Job drawing, mm, ordinate dimensions from the low corner. One solid piece. A direction names the side the tool comes from. Coordinates: 2 decimals unless noted, no trailing zeros. Order: outer loops, then holes, each group sorted by start corner. A loop starts at its lowest first (then second) coordinate and runs counter-clockwise, first axis right, second up. Notation, with made-up numbers: (-21, 52) -> (1, 52) arc R16 ccw to (1, 83) -> close; hole circle Ø3 at (66, 41.5). An arc over 180 degrees is marked (long way). Use CSV: the item, a comma, the result in double quotes. Start each with the question number.
(1) Tool access for the marked faces 4 and 5: list every direction of +Z, -Z, +X, -X, +Y, -Y with a clear straight run to the whole face (end or side of a thin tool).
(2) Cut at C-C on y = 14. Write the cut outline in (x, z).
(3) Cut at A-A on y = 3.75. Write the cut outline in (x, z), plus the area to 3 significant figures.
(4) Cut at D-D on z = 20. Write the cut outline in (x, y).
(5) Pin check, flat tips, straight feed: pin 1 Ø8 at (x, y) = (7.5, 9) entering from +Z; pin 2 Ø1.6 at (x, z) = (33, 13) entering from +Y; pin 3 Ø2.5 at (x, z) = (6, 27) entering from +Y; pin 4 Ø8 at (y, z) = (3, 30.5) entering from -X (1 decimal). Stop position of each tip, or through.
(6) Pull direction X, two halves, no side cores. Call the marked faces 1, 2 and 3: pulls with the +X half, pulls with the -X half, needs draft (parallel to the pull), parting line crosses it, or undercut.
(7) Cut at B-B on z = 13. Write the cut outline in (x, y) (1 decimal).
(8) Probe L1, parallel to X at y = 3, z = 27 (1 decimal); L2, parallel to X at y = 5.5, z = 27 (1 decimal); L3, parallel to X at y = 13.3, z = 13 (1 decimal). List the from-to ranges inside material, lowest first.
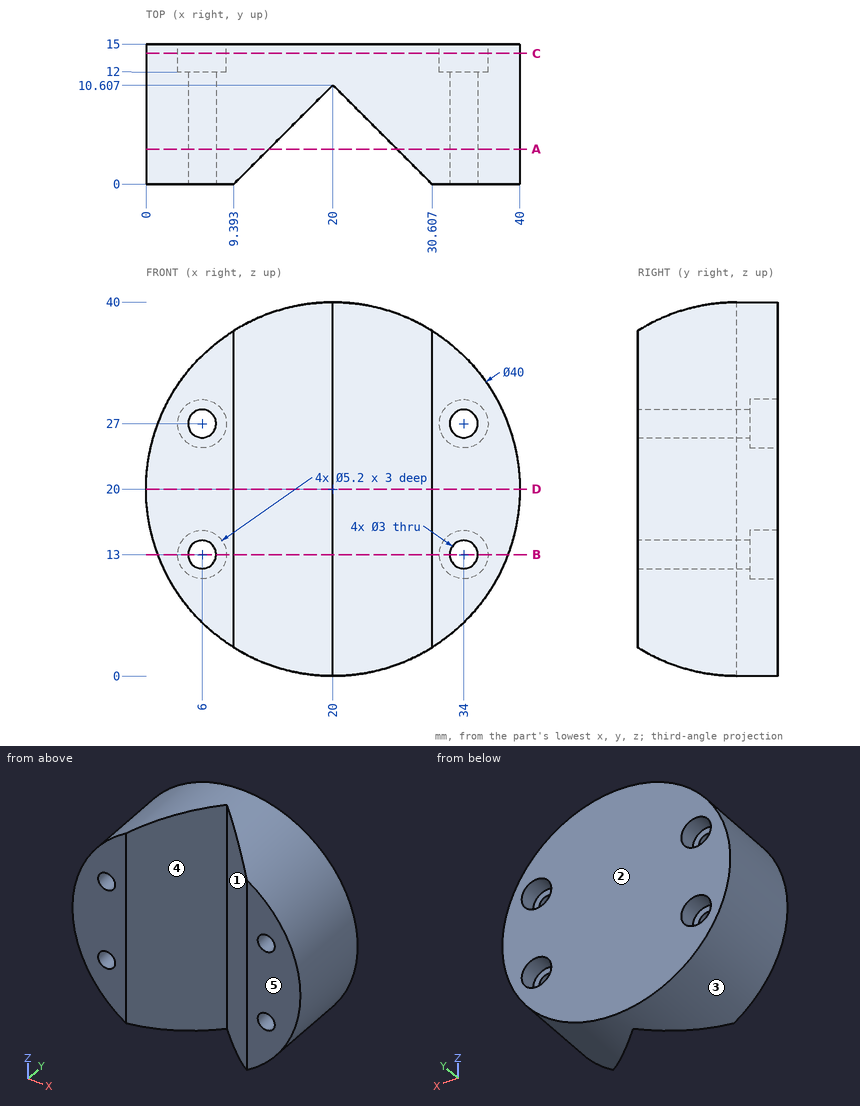
Outcome:
1,face 4,"+Z, -Z, -Y"
1,face 5,"+Z, -Z, +X, -X, -Y"
2,outline,"circle Ø40 at (20, 20); hole circle Ø5.2 at (6, 13); hole circle Ø5.2 at (6, 27); hole circle Ø5.2 at (34, 13); hole circle Ø5.2 at (34, 27)"
3,outline,"(13.14, 1.21) -> (13.14, 38.79) arc R20 ccw to start; (26.86, 1.21) arc R20 ccw to (26.86, 38.79) -> close; hole circle Ø3 at (6, 13); hole circle Ø3 at (6, 27); hole circle Ø3 at (34, 13); hole circle Ø3 at (34, 27)"
3,area,"691 mm2"
4,outline,"(0, 0) -> (9.39, 0) -> (20, 10.61) -> (30.61, 0) -> (40, 0) -> (40, 15) -> (0, 15) -> close"
5,pin 1,"z = 38.1"
5,pin 2,"y = 12"
5,pin 3,"through"
5,pin 4,"x = 1.1"
6,face 1,"undercut"
6,face 2,"needs draft"
6,face 3,"parting line crosses it"
7,outline,"(1.3, 0) -> (4.5, 0) -> (4.5, 12) -> (3.4, 12) -> (3.4, 15) -> (1.3, 15) -> close; (7.5, 0) -> (9.4, 0) -> (20, 10.6) -> (30.6, 0) -> (32.5, 0) -> (32.5, 12) -> (31.4, 12) -> (31.4, 15) -> (8.6, 15) -> (8.6, 12) -> (7.5, 12) -> close; (35.5, 0) -> (38.7, 0) -> (38.7, 15) -> (36.6, 15) -> (36.6, 12) -> (35.5, 12) -> close"
8,L1,"1.3 to 4.5, 7.5 to 12.4, 27.6 to 32.5, 35.5 to 38.7"
8,L2,"1.3 to 4.5, 7.5 to 14.9, 25.1 to 32.5, 35.5 to 38.7"
8,L3,"1.3 to 3.4, 8.6 to 31.4, 36.6 to 38.7"
